The listing builds one solid part. Answer for the finished solid, in the listing's coordinates (mm). Face numbers are marked on the shaded views. A direction names the side the tool comes from. Give positions to 0.01 mm unless a question says otherwise; leave off trailing zeros. Write each loop counter-clockwise with the first axis right and the second up, starting at its lowest first coordinate (ties: lowest second). Pieces come first, ordered by that corner, then holes.
```python
from build123d import *
from build123d.topology import SkipClean

# Parameters (mm, degrees)
SKETCH1_R               = 7
BOSS_EXTRUDE1_DEPTH     = 16
BOSS_EXTRUDE2_START     = -3
SKETCH3_R               = 7
BOSS_EXTRUDE2_DEPTH     = 3
CUT_EXTRUDE1_DEPTH      = 39.354433
CUT_EXTRUDE1_DEPTH_BACK = 39.354433
SKETCH2_R               = 3
BOSS_EXTRUDE3_START     = -6
BOSS_EXTRUDE3_DEPTH     = 6
BOSS_EXTRUDE4_START     = -16
BOSS_EXTRUDE4_DEPTH     = 16
BOSS_EXTRUDE5_START     = -21
BOSS_EXTRUDE5_DEPTH     = 21
CUT_EXTRUDE2_DEPTH      = 5
CUT_EXTRUDE3_START      = -21
CUT_EXTRUDE3_DEPTH      = 5
CUT_EXTRUDE4_DEPTH      = 67.585002
CUT_EXTRUDE4_DEPTH_BACK = 67.585002
SKETCH6_R               = 3.25


with BuildPart() as part:
    # Sketch1 → Boss-Extrude1 (new body)
    with BuildSketch(Plane.XY):
        with BuildLine():
            ThreePointArc((16.808917, -9.124391), (14.337584, -12.994121), (10, -14.5))
            Line((10, -14.5), (15, -14.5))
            Line((15, -14.5), (15, -17.75))
            Line((15, -17.75), (30, -17.75))
            Line((30, -17.75), (30, -14.75))
            Line((30, -14.75), (16.808917, -9.124391))
        make_face()
        with Locations((10, -7.5)):
            Circle(SKETCH1_R)
        with BuildLine():
            Line((0, -10), (3.461652, -10))
            ThreePointArc((3.461652, -10), (3, -7.5), (3.461652, -5))
            Line((3.461652, -5), (0, -5))
            Line((0, -5), (0, -10))
        make_face()
    extrude(amount=BOSS_EXTRUDE1_DEPTH)

    # Sketch3 → Boss-Extrude2 (add)
    with BuildSketch(Plane.XY.offset(BOSS_EXTRUDE2_START)):
        with Locations(Location((10, -7.5, 0), (0, 0, 159.075168))):
            Circle(SKETCH3_R)
    extrude(amount=BOSS_EXTRUDE2_DEPTH)

    # Sketch2 → Cut-Extrude1 (cut, two sides: drawn at the far end of the back side and taken through both)
    with BuildSketch(Plane.XY.offset(-CUT_EXTRUDE1_DEPTH_BACK)):
        with Locations((10, -7.5)):
            Circle(SKETCH2_R)
        with BuildLine():
            ThreePointArc((12.752773, -6.307423), (12.937543, -6.891034), (13, -7.5))
            Line((13, -7.5), (16.959704, -9.188697))
            Line((16.959704, -9.188697), (17.35199, -8.268854))
            Line((17.35199, -8.268854), (12.752773, -6.307423))
        make_face()
    extrude(amount=CUT_EXTRUDE1_DEPTH + CUT_EXTRUDE1_DEPTH_BACK, mode=Mode.SUBTRACT)

    # Sketch4 → Boss-Extrude3 (add)
    with BuildSketch(Plane.XY.offset(16).offset(BOSS_EXTRUDE3_START)):
        with BuildLine():
            Line((12.202752, -0.855613), (7.5, 37.25))
            Line((7.5, 37.25), (7.5, -0.961652))
            ThreePointArc((7.5, -0.961652), (9.842202, -0.501779), (12.202752, -0.855613))
        make_face()
    extrude(amount=BOSS_EXTRUDE3_DEPTH)

    # Sketch4<6> → Boss-Extrude4 (add)
    with BuildSketch(Plane.XY.offset(16).offset(BOSS_EXTRUDE4_START)):
        with BuildLine():
            Line((7.5, 37.25), (7.5, 40.635622))
            ThreePointArc((7.5, 40.635622), (4.114378, 38.135622), (0, 37.25))
            Line((0, 37.25), (0, 32.25))
            ThreePointArc((0, 32.25), (1.767767, 31.517767), (2.5, 29.75))
            Line((2.5, 29.75), (2.5, -2.5))
            ThreePointArc((2.5, -2.5), (1.767767, -4.267767), (0, -5))
            Line((0, -5), (3.461652, -5))
            ThreePointArc((3.461652, -5), (5.050253, -2.550253), (7.5, -0.961652))
            Line((7.5, -0.961652), (7.5, 37.25))
        make_face()
    extrude(amount=BOSS_EXTRUDE4_DEPTH)

    # Sketch4<7> → Boss-Extrude5 (add)
    with BuildSketch(Plane.XY.offset(16).offset(BOSS_EXTRUDE5_START)):
        with BuildLine():
            ThreePointArc((0, 37.25), (4.114378, 38.135622), (7.5, 40.635622))
            ThreePointArc((7.5, 40.635622), (9.114378, 51.364378), (0, 57.25))
            Line((0, 57.25), (0, 49.65))
            ThreePointArc((0, 49.65), (2.4, 47.25), (0, 44.85))
            Line((0, 44.85), (0, 37.25))
        make_face()
    extrude(amount=BOSS_EXTRUDE5_DEPTH)

    # Mirror1: part across plane


with BuildPart() as part_1:
    with SkipClean():  # the faces are left unmerged after this step: merging them gives an invalid solid
        add(part.part)
        add(part.part.mirror(Plane(origin=(0, 0, 0), x_dir=(0, 0, 1), z_dir=(1, 0, 0))))

    # Sketch5 → Cut-Extrude2 (cut)
    with SkipClean():  # the faces are left unmerged after this step: merging them gives an invalid solid
        with BuildSketch(Plane.XY.offset(16)):
            Polygon((4.25, 49.703739), (0, 52.157477), (-4.25, 49.703739), (-4.25, 44.796261), (0, 42.342523), (4.25, 44.796261), align=None)
        extrude(amount=-CUT_EXTRUDE2_DEPTH, mode=Mode.SUBTRACT)

    # Sketch5<2> → Cut-Extrude3 (cut)
    with SkipClean():  # the faces are left unmerged after this step: merging them gives an invalid solid
        with BuildSketch(Plane.XY.offset(16).offset(CUT_EXTRUDE3_START)):
            Polygon((4.25, 49.703739), (0, 52.157477), (-4.25, 49.703739), (-4.25, 44.796261), (0, 42.342523), (4.25, 44.796261), align=None)
        extrude(amount=CUT_EXTRUDE3_DEPTH, mode=Mode.SUBTRACT)

    # Sketch6 → Cut-Extrude4 (cut, two sides: drawn at the far end of the back side and taken through both)
    with SkipClean():  # the faces are left unmerged after this step: merging them gives an invalid solid
        with BuildSketch(Plane.XY.offset(11).offset(-CUT_EXTRUDE4_DEPTH_BACK)):
            with Locations((0, 47.25)):
                Circle(SKETCH6_R)
        extrude(amount=CUT_EXTRUDE4_DEPTH + CUT_EXTRUDE4_DEPTH_BACK, mode=Mode.SUBTRACT)


solid = part_1.part
```
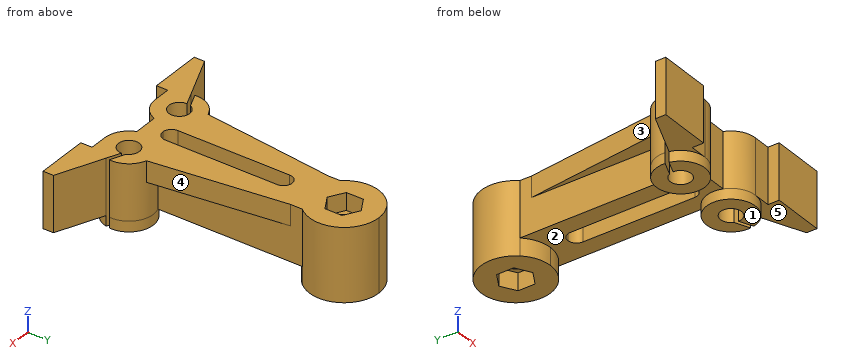
Item 1: Each of these flat-tipped pins is pushed along its axis until it touches: P1, Ø12, axis at y = 42.5, z = -0.5, coming from the -X side; P2, Ø5, axis at y = 14.5, z = 7, coming from the +X side; P3, Ø7.5, axis at x = 3, y = 23.5, coming from the -Z side. Where does it stop, or does it pass through?
Conclusion:
P1: stops at x = -10
P2: stops at x = 7.5
P3: stops at z = 0
Item 2: A cutting plane is placed at B-B, the plane z = 12.5. Count the separate pieces of the cut face and the enclosed holes in it, plus the area to 3 significant figures.
Conclusion:
separate pieces: 1
enclosed holes: 2
area: 1,330 mm2
Item 3: A cutting plane is placed at A-A, the plane y = 47.25. Give the vertices of the cut face in (x, z).
Conclusion:
outline: (-10, -5) - (-4.25, -5) - (-4.25, 0) - (-3.25, 0) - (-3.25, 11) - (-4.25, 11) - (-4.25, 16) - (-10, 16) - close; (3.25, 0) - (4.25, 0) - (4.25, -5) - (10, -5) - (10, 16) - (4.25, 16) - (4.25, 11) - (3.25, 11) - close
Item 4: A cutting plane is placed at D-D, the plane x = -20.5. Give the vertices of the cut face in (y, z), plus the area to 3 significant figures.
Conclusion:
outline: (-17.75, 0) - (-10.7, 0) - (-10.7, 16) - (-17.75, 16) - close
area: 113 mm2
Item 5: Which of the six approach directions +Z, -Z, +X, -X, +Y, -Y give full straight-line access (tool end or side, diameter ignored) to the marked faces 1, 2, 3, 4 and 5?
Conclusion:
face 1: -Z, +X, -X, -Y
face 2: -Z
face 3: +Z, -Z, -X
face 4: +Z, -Z, +X
face 5: -Z, +X, -Y
Item 6: Consider probe 1 along Y at (x, z) = (0, 6.25); probe 2 along X at (y, z) = (5.5, 6.75); probe 3 along X at (y, z) = (47.25, 7.25). Determine where each line is inside the solid, lowest interval first.
Conclusion:
probe 1: y = -10 to -5, 32.25 to 44, 50.5 to 57.25
probe 2: x = -7.5 to -2.5, 2.5 to 7.5
probe 3: x = -10 to -3.25, 3.25 to 10
Item 7: A cutting plane is placed at C-C, the plane y = 1.5. Give the vertices of the cut face in (x, z).
Conclusion:
outline: (-11.91, 10) - (-7.5, 10) - (-7.5, 0) - (-2.5, 0) - (-2.5, 16) - (-11.91, 16) - close; (2.5, 0) - (7.5, 0) - (7.5, 10) - (11.91, 10) - (11.91, 16) - (2.5, 16) - close
